Source: CAD feature listing. Evaluate the final solid. Frame: model axes, mm. Face numbers are marked on the shaded views. A direction names the side the tool comes from. Round coordinates to 2 decimals unless told otherwise and drop trailing zeros. Write each loop counter-clockwise with the first axis right and the second up, starting at its lowest first coordinate (ties: lowest second). Pieces come first, ordered by that corner, then holes.
Autodesk Fusion 360 part; units mm, degrees
sketch "Sketch4" plane through (0, 0, 0) normal (0, 0, 1) x (1, 0, 0)
  line L0 (-14, 13) -> (26, 13)
  line L1 (26, 13) -> (26, -27)
  line L2 (26, -27) -> (-14, -27)
  line L3 (-14, -27) -> (-14, 13)
  line L4 (6, 11) -> (11.7842, -0.4932)
  line L5 (11.7842, -0.4932) -> (24.8229, -2.4867)
  line L6 (24.8229, -2.4867) -> (15.448, -11.6461)
  line L7 (15.448, -11.6461) -> (18, -25)
  line L8 (18, -25) -> (6, -19)
  line L9 (6, -19) -> (-5.9959, -25.493)
  line L10 (-5.9959, -25.493) -> (-3.6252, -12.5082)
  line L11 (-3.6252, -12.5082) -> (-13, -3)
  line L12 (-13, -3) -> (0.0021, -0.4393)
  line L13 (0.0021, -0.4393) -> (6, 11)
extrude "Extrude1" add sketch "Sketch4" along normal blind 3 contours L4 L5 L6 L7 L8 L9 L10 L11 L12 L13
cylinder "CylinderPrimitive1" cut diameter 2.33 height -3 placed x (1, 0, 0) y (0, 1, 0) z (0, 0, 1) at (5.6258, 2.3767, 3)
sketch "Sketch2" plane through (0, 0, 0) normal (0, 0, 1) x (1, 0, 0)
  line L0 (-22.5492, 19.9652) -> (17.4508, 19.9652)
  line L1 (17.4508, 19.9652) -> (17.4508, -20.0348)
  line L2 (17.4508, -20.0348) -> (-22.5492, -20.0348)
  line L3 (-22.5492, -20.0348) -> (-22.5492, 19.9652)
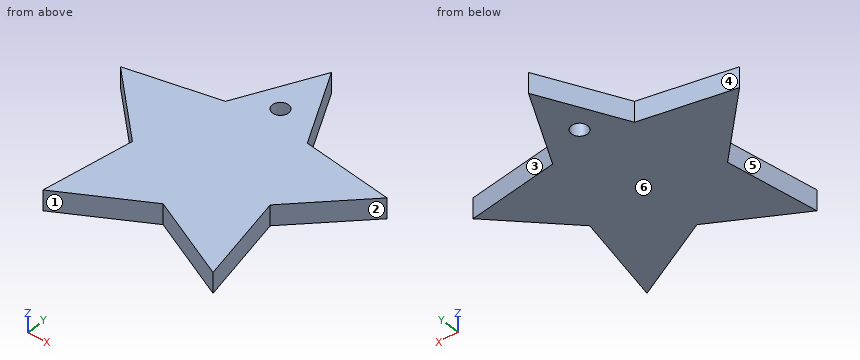
1) Section query C-C on z = 1.6. Return the cut outline in (x, y) (3 decimals).
Taken from the geometry:
outline: (-13, -3) - (-3.625, -12.508) - (-5.996, -25.493) - (6, -19) - (18, -25) - (15.448, -11.646) - (24.823, -2.487) - (11.784, -0.493) - (6, 11) - (0.002, -0.439) - close; hole circle Ø2.33 at (5.626, 2.377)
2) Pull-direction query (Y, two-part tool) for the marked faces 4, 5 and 6; classes: released by +Y, released by -Y, zero draft, split by the parting line, or undercut.
Taken from the geometry:
face 4: released by +Y
face 5: undercut
face 6: zero draft
3) Contact query for flat-ended pins moving along their axis: P1, Ø1.4, axis at x = 5.63, y = 2.38, coming from the +Z side; P2, Ø10, axis at x = -0.5, y = -3.5, coming from the -Z side. Output: stop coordinate, or through.
Taken from the geometry:
P1: passes through
P2: stops at z = 0
4) Section query A-A on x = 17. Return the cut outline in (y, z), then the cut area to 3 significant figures.
Taken from the geometry:
outline: (-24.5, 0) - (-19.77, 0) - (-19.77, 3) - (-24.5, 3) - close; (-10.13, 0) - (-1.29, 0) - (-1.29, 3) - (-10.13, 3) - close
area: 40.7 mm2
5) Section query B-B on y = -20. Return the cut outline in (x, z).
Taken from the geometry:
outline: (-4.99, 0) - (4.15, 0) - (4.15, 3) - (-4.99, 3) - close; (8, 0) - (17.04, 0) - (17.04, 3) - (8, 3) - close
6) Reachability of the marked faces 1, 2 and 3 from +Z, -Z, +X, -X, +Y, -Y: full face, straight path, thin tool, end or side. Return the list, or none.
Taken from the geometry:
face 1: +Z, -Z, -Y
face 2: +Z, -Z, +X
face 3: +Z, -Z, +X, +Y
7) Material intervals for line 1 (X direction, y = 1.5, z = 2.8); line 2 (Y direction, x = 22, z = 0.5); line 3 (Y direction, x = 6.5, z = 0.4), sorted ascending.
Taken from the geometry:
line 1: x = 1.02 to 4.86, 6.39 to 10.78
line 2: y = -5.24 to -2.06
line 3: y = -19.25 to 1.61, 3.15 to 10.01
8) Section query D-D on x = 4. Return the cut outline in (y, z).
Taken from the geometry:
outline: (-20.08, 0) - (7.19, 0) - (7.19, 3) - (-20.08, 3) - close
